Read the model definition and answer for the solid it produces. Units are mm, in the model's axes. A direction names the side the tool comes from. Coordinates: 2 decimals unless noted, no trailing zeros. Loops run counter-clockwise (first coordinate to the right, second up) from the corner with the lowest first, then second, coordinate; pieces in that order, holes last. Notation, with made-up numbers: (13.5, 72) -> (63.5, 72) arc R25 ccw to (63.5, 95) -> close; hole circle Ø10 at (25, -25.5). An arc over 180 degrees is marked (long way). Answer as a JSON object with one key per item and string values. Group by question number.
Q1. For faces 4 (the cylindrical face through (-20.745, 20.861, 24.157)), 5 (the cylindrical face through (19.43, 19.35, 25.17)), determine the directions among +Z, -Z, +X, -X, +Y, -Y from which every point of the face is accessible in a straight line to the end or side of a thin tool.
Q2. Straight lines are drawn through the part: line 1 along X through (y, z) = (-1, 32.5); line 2 along Z through (x, y) = (15, 18). For each, find the intervals that lie inside material, in ascending order. Write a range as [from, to].
Q3. Determine the mould class of faces 1 (the flat face through (-23, 0, 24)), 2 (the cylindrical face through (20.861, 20.745, 24.157)), 3 (the cylindrical face through (-19.35, 19.43, 25.17)) for opening direction Y: released by +Y, released by -Y, zero draft, split by the parting line, or undercut.
Q4. The part is cut by section B-B on y = -14.5. Write down the section's boundary in (x, z), and give its area (3 significant figures).
Q5. The part is cut by section A-A on z = 36.5. Write down the section's boundary in (x, y).
from build123d import *

# Parameters (mm, degrees)
SKETCH1_W           = 42
SKETCH1_H           = 42
BOSS_EXTRUDE1_DEPTH = 2
FILLET1_R           = 5.5
BOSS_EXTRUDE2_DEPTH = 49


with BuildPart() as part:
    # Sketch1 → Boss-Extrude1 (new body)
    with BuildSketch(Plane.XY):
        Rectangle(SKETCH1_W, SKETCH1_H)
    extrude(amount=BOSS_EXTRUDE1_DEPTH)

    # Fillet1
    fillet1_edges = [part.edges().sort_by_distance(p)[0] for p in [
        (-21, 21, 1),
        (21, 21, 1),
        (21, -21, 1),
        (-21, -21, 1),
    ]]
    fillet(fillet1_edges, radius=FILLET1_R)

    # Sketch2 → Boss-Extrude2 (add)
    with BuildSketch(Plane.XY):
        with BuildLine():
            Line((-23, 15.5), (-23, -15.5))
            ThreePointArc((-23, -15.5), (-20.803300859, -20.803300859), (-15.5, -23))
            Line((-15.5, -23), (15.5, -23))
            ThreePointArc((15.5, -23), (20.803300859, -20.803300859), (23, -15.5))
            Line((23, -15.5), (23, 15.5))
            ThreePointArc((23, 15.5), (20.803300859, 20.803300859), (15.5, 23))
            Line((15.5, 23), (-15.5, 23))
            ThreePointArc((-15.5, 23), (-20.803300859, 20.803300859), (-23, 15.5))
        make_face()
        with BuildLine():
            Line((-21, 15.5), (-21, -15.5))
            ThreePointArc((-21, -15.5), (-19.389087297, -19.389087297), (-15.5, -21))
            Line((-15.5, -21), (15.5, -21))
            ThreePointArc((15.5, -21), (19.389087297, -19.389087297), (21, -15.5))
            Line((21, -15.5), (21, 15.5))
            ThreePointArc((21, 15.5), (19.389087297, 19.389087297), (15.5, 21))
            Line((15.5, 21), (-15.5, 21))
            ThreePointArc((-15.5, 21), (-19.389087297, 19.389087297), (-21, 15.5))
        make_face(mode=Mode.SUBTRACT)
    extrude(amount=BOSS_EXTRUDE2_DEPTH)


solid = part.part
Final values:
{
 "1": {"face 4": "+Z, -Z, -X, +Y", "face 5": "+Z"},
 "2": {"line 1": "x = [-23, -21], [21, 23]", "line 2": "z = [0, 2]"},
 "3": {"face 1": "zero draft", "face 2": "released by +Y", "face 3": "undercut"},
 "4": {"outline": "(-23, 0) -> (23, 0) -> (23, 49) -> (21, 49) -> (21, 2) -> (-21, 2) -> (-21, 49) -> (-23, 49) -> close", "area": "280 mm2"},
 "5": {"outline": "(-23, -15.5) arc R7.5 ccw to (-15.5, -23) -> (15.5, -23) arc R7.5 ccw to (23, -15.5) -> (23, 15.5) arc R7.5 ccw to (15.5, 23) -> (-15.5, 23) arc R7.5 ccw to (-23, 15.5) -> close; hole (-21, -15.5) arc R5.5 ccw to (-15.5, -21) -> (15.5, -21) arc R5.5 ccw to (21, -15.5) -> (21, 15.5) arc R5.5 ccw to (15.5, 21) -> (-15.5, 21) arc R5.5 ccw to (-21, 15.5) -> close"}
}
